```python
from build123d import *

# Parameters (mm, degrees)
CROQUIS1_W              = 80.8
CROQUIS1_H              = 25
CROQUIS1_R              = 1.5
SALIENTE_EXTRUIR1_DEPTH = 5
CROQUIS1_3_W            = 80.8
CROQUIS1_3_H            = 5
SALIENTE_EXTRUIR2_DEPTH = 26
CROQUIS1_4_R            = 1.5
SALIENTE_EXTRUIR3_DEPTH = 5
SALIENTE_EXTRUIR4_DEPTH = 26
CROQUIS3_R              = 2.25
CORTAR_EXTRUIR1_DEPTH   = 26
SALIENTE_EXTRUIR5_DEPTH = 21
CORTAR_EXTRUIR2_DEPTH   = 21
CROQUIS6_W              = 37.983880197
CROQUIS6_H              = 26
CORTAR_EXTRUIR3_DEPTH   = 120
CROQUIS7_W              = 35
CROQUIS7_H              = 26
SALIENTE_EXTRUIR6_DEPTH = 0.5


with BuildPart() as part:
    # Croquis1 → Saliente-Extruir1 (new body)
    with BuildSketch(Plane(origin=(0, 0, 0), x_dir=(1, 0, 0), z_dir=(0, 1, 0))):
        with Locations((0, -10)):
            Rectangle(CROQUIS1_W, CROQUIS1_H)
        with Locations((15.4, -12.5)):
            Circle(CROQUIS1_R, mode=Mode.SUBTRACT)
        with Locations((-15.4, -12.5)):
            Circle(CROQUIS1_R, mode=Mode.SUBTRACT)
    extrude(amount=SALIENTE_EXTRUIR1_DEPTH)

    # Croquis1_3 → Saliente-Extruir2 (add)
    with BuildSketch(Plane(origin=(0, 0, 0), x_dir=(1, 0, 0), z_dir=(0, 1, 0))):
        Rectangle(CROQUIS1_3_W, CROQUIS1_3_H)
    extrude(amount=SALIENTE_EXTRUIR2_DEPTH)

    # Croquis1_4 → Saliente-Extruir3 (add)
    with BuildSketch(Plane(origin=(0, 0, 0), x_dir=(1, 0, 0), z_dir=(0, 1, 0))):
        Polygon((-45.4, -2.5), (-40.4, -2.5), (-40.4, 2.5), (-40.4, 37.5), (-45.4, 37.5), align=None)
        Polygon((-40.4, -22.5), (-40.4, -2.5), (-45.4, -2.5), (-45.4, 37.5), (-66.4, 37.5), (-66.4, -22.5), align=None)
        with Locations((-55.4, 12.5)):
            Circle(CROQUIS1_4_R, mode=Mode.SUBTRACT)
        Polygon((45.4, -2.5), (40.4, -2.5), (40.4, -22.5), (66.4, -22.5), (66.4, 37.5), (45.4, 37.5), align=None)
        with Locations((55.4, 12.5)):
            Circle(CROQUIS1_4_R, mode=Mode.SUBTRACT)
        Polygon((40.4, 2.5), (40.4, -2.5), (45.4, -2.5), (45.4, 37.5), (40.4, 37.5), align=None)
    extrude(amount=SALIENTE_EXTRUIR3_DEPTH)

    # Croquis1_5 → Saliente-Extruir4 (add)
    with BuildSketch(Plane(origin=(0, 0, 0), x_dir=(1, 0, 0), z_dir=(0, 1, 0))):
        Polygon((-45.4, -2.5), (-40.4, -2.5), (-40.4, 2.5), (-40.4, 37.5), (-45.4, 37.5), align=None)
        Polygon((40.4, 2.5), (40.4, -2.5), (45.4, -2.5), (45.4, 37.5), (40.4, 37.5), align=None)
    extrude(amount=SALIENTE_EXTRUIR4_DEPTH)

    # Croquis3 → Cortar-Extruir1 (cut)
    with BuildSketch(Plane.XY.offset(2.5)):
        with Locations((-24, 10)):
            Circle(CROQUIS3_R)
        with Locations((23.5, 10)):
            Circle(CROQUIS3_R)
    extrude(amount=-CORTAR_EXTRUIR1_DEPTH, mode=Mode.SUBTRACT)

    # Croquis4 → Saliente-Extruir5 (add)
    with BuildSketch(Plane(origin=(0, 5, 0), x_dir=(1, 0, 0), z_dir=(0, 1, 0))):
        Polygon((-45.4, -0.5), (-45.4, -2.5), (-43.4, -2.5), (-64.4, -22.5), (-66.4, -22.5), (-66.4, -20.5), align=None)
    saliente_extruir5 = extrude(amount=SALIENTE_EXTRUIR5_DEPTH)

    # Croquis5 → Cortar-Extruir2 (cut)
    with BuildSketch(Plane(origin=(-19.393579073, 0, -20.363258026), x_dir=(0.724137931, 0, -0.689655172), z_dir=(0.689655172, 0, 0.724137931))):
        Polygon((-62.151724138, 5), (-33.151724138, 26), (-26.486949689, 30.82621598), (-82.759555013, 33.403814281), (-84.060607683, 5), align=None)
    cortar_extruir2 = extrude(amount=-CORTAR_EXTRUIR2_DEPTH, mode=Mode.SUBTRACT)

    # Simetr_a1: Saliente-Extruir5 across plane
    add(saliente_extruir5.mirror(Plane(origin=(0, 0, 0), x_dir=(0, 0, 1), z_dir=(1, 0, 0))))

    # Simetr_a2: Cortar-Extruir2 across plane
    add(cortar_extruir2.mirror(Plane(origin=(0, 0, 0), x_dir=(0, 0, 1), z_dir=(1, 0, 0))), mode=Mode.SUBTRACT)

    # Croquis6 → Cortar-Extruir3 (cut)
    with BuildSketch(Plane(origin=(0, 0, -37.5), x_dir=(-1, 0, 0), z_dir=(0, 0, -1))):
        with Locations((59.391940099, 13)):
            Rectangle(CROQUIS6_W, CROQUIS6_H)
    extrude(amount=-CORTAR_EXTRUIR3_DEPTH, mode=Mode.SUBTRACT)

    # Croquis7 → Saliente-Extruir6 (add)
    with BuildSketch(Plane.ZY.offset(-40.4)):
        with Locations((-20, 13)):
            Rectangle(CROQUIS7_W, CROQUIS7_H)
    extrude(amount=SALIENTE_EXTRUIR6_DEPTH)


solid = part.part
```
Geometry: final body of the model. Coordinates: model frame, mm. A direction names the side the tool comes from. Give positions to 0.01 mm unless a question says otherwise; leave off trailing zeros. Loops run counter-clockwise (first coordinate to the right, second up) from the corner with the lowest first, then second, coordinate; pieces in that order, holes last. Notation, with made-up numbers: (36, 2.5) - (93, 2.5) arc R17 cw to (93, 7.5) - close; hole circle Ø9 at (60, 57.25). An arc over 180 degrees is marked (long way). Answer as CSV lines item,"result". Start each with the question number.
(1) Section query D-D (z = 12.5). Output: boundary loops of the cut face in (x, y), and give its area (3 significant figures).
(2) Pin query (flat end, axial travel): P1, Ø6.5, axis at x = 3, y = 19.5, coming from the +Z side; P2, Ø10.5, axis at y = 11.5, z = -12, coming from the +X side; P3, Ø2, axis at y = 8, z = 14.5, coming from the +X side. Return the tip coordinate at first contact, or that it passes through.
(3) Section query A-A (x = 15.4). Output: boundary loops of the cut face in (y, z).
(4) Ray query, line 1 along Y through (x, z) = (-24, -1); line 2 along Z through (x, y) = (-15.4, 3.45); line 3 along Z through (x, y) = (55.4, 2.6). Return the intervals inside material, ascending. Write a range as [from, to].
(5) Section query C-C (y = 10). Output: boundary loops of the cut face in (x, z).
(6) Mould query, pull axis X, two halves, no side actions, for faces 6 (the face through (66.4, 2, -7)), 7 (the face through (-1, 13, -2.5)), 8 (the face through (-21.854, 10.676, 0.035)). Classes: +X half, -X half, draft (parallel to the pull), parting line (faces both ways), or undercut.
(7) Reachability of faces 1 (the face through (25.646, 10.676, 0.035)), 2 (the face through (51.366, 10.673, 6.182)), 3 (the face through (39.9, 13, -20)), 4 (the face through (51.42, 13.02, 10.14)), 5 (the face through (56.83, 2.46, -12.95)) from +Z, -Z, +X, -X, +Y, -Y: full face, straight path, thin tool, end or side. Return the list, or none.
(8) Section query B-B (z = -12.5). Output: boundary loops of the cut face in (x, y).
Worked answers:
1,outline,"(-40.4, 0) - (-16.9, 0) - (-16.9, 5) - (-40.4, 5) - close; (-13.9, 0) - (13.9, 0) - (13.9, 5) - (-13.9, 5) - close; (16.9, 0) - (66.4, 0) - (66.4, 5) - (58, 5) - (58, 13.35) - (53.9, 15.5) - (53.9, 5) - (16.9, 5) - close"
1,area,"543 mm^2"
2,P1,"stops at z = 2.5"
2,P2,"stops at x = 45.4"
2,P3,"stops at x = 61.15"
3,outline,"(0, -2.5) - (26, -2.5) - (26, 2.5) - (5, 2.5) - (5, 11) - (0, 11) - close; (0, 14) - (5, 14) - (5, 22.5) - (0, 22.5) - close"
4,line 1,"y = [0, 7.75], [12.25, 26]"
4,line 2,"z = [-2.5, 11], [14, 22.5]"
4,line 3,"z = [-37.5, -14], [-11, 22.5]"
5,outline,"(-40.4, -2.5) - (-26.25, -2.5) - (-26.25, 2.5) - (-40.4, 2.5) - close; (-21.75, -2.5) - (21.25, -2.5) - (21.25, 2.5) - (-21.75, 2.5) - close; (25.75, -2.5) - (39.9, -2.5) - (39.9, -37.5) - (45.4, -37.5) - (45.4, 0.5) - (61.35, 15.69) - (59.4, 17.74) - (43.4, 2.5) - (25.75, 2.5) - close"
6,face 6,"+X half"
6,face 7,"draft"
6,face 8,"undercut"
7,face 1,"+Z, -Z"
7,face 2,"-Z, +X, +Y"
7,face 3,"-Z, -X, +Y, -Y"
7,face 4,"+Z, -X, +Y"
7,face 5,"+Y, -Y"
8,outline,"(39.9, 0) - (53.9, 0) - (53.9, 5) - (45.4, 5) - (45.4, 26) - (39.9, 26) - close; (56.9, 0) - (66.4, 0) - (66.4, 5) - (56.9, 5) - close"
